The model under review builds one solid part; all positions refer to its coordinate system, in mm. A direction names the side the tool comes from. Coordinates: 2 decimals unless noted, no trailing zeros. Order: outer loops, then holes, each group sorted by start corner. A loop starts at its lowest first (then second) coordinate and runs counter-clockwise, first axis right, second up. Notation, with made-up numbers: M 81,-33.5 L 102,-33.5 A33 cw 102,-4.5 Z; hole C 6.5,67 d4. An arc over 180 degrees is marked long. Answer in a Markdown table with one row per item.
Solid Edge part; units mm, degrees
sketch "Sketch1" plane through (0, 0, 0) normal (0, -1, 0) x (1, 0, 0)
  line L0 (5.1, 0) -> (5.1, 1.5)
  line L1 (5.1, 1.5) -> (11, 1.5)
  line L2 (11, 1.5) -> (11, 5)
  line L3 (11, 5) -> (5.1, 5)
  line L4 (5.1, 5) -> (5.1, 15)
  line L5 (5.1, 15) -> (4, 15)
  line L6 (4, 15) -> (4, 0)
  line L7 (4, 0) -> (5.1, 0)
  dimension "D1" = 5.1
  dimension "D2" = 11
  dimension "D3" = 5.1
revolve "RevolvedProtrusion1" add sketch "Sketch1" angle 360 about axis through (0, 0, 0) along (0, 0, 1)
sketch "Sketch2" plane through (0, 0, 5) normal (0, 0, 1) x (1, 0, 0)
  circle A0 centre (0, 8) radius 1.6
  circle A1 centre (8, 0) radius 1.6
  circle A2 centre (0, -8) radius 1.6
  circle A3 centre (-8, 0) radius 1.6
extrude "Cutout1" cut sketch "Sketch2" against normal through all
chamfer "Chamfer1" distance 0.4 angle 45 2 edges at (-5.1, 0, 15) (-5.1, 0, 0)
(1) Take a section at A-A (x = 0). Write out the cut boundary in (y, z), then the cut area to 3 significant figures.
Report:
| item | result |
|---|---|
| outline | M -11,1.5 L -9.6,1.5 L -9.6,5 L -11,5 Z; M -6.4,1.5 L -5.1,1.5 L -5.1,0.4 L -4.7,0 L -4,0 L -4,15 L -4.7,15 L -5.1,14.6 L -5.1,5 L -6.4,5 Z; M 4,0 L 4.7,0 L 5.1,0.4 L 5.1,1.5 L 6.4,1.5 L 6.4,5 L 5.1,5 L 5.1,14.6 L 4.7,15 L 4,15 Z; M 9.6,1.5 L 11,1.5 L 11,5 L 9.6,5 Z |
| area | 51.6 mm^2 |
(2) Take a section at D-D (y = 8). Write out the cut boundary in (x, z).
Report:
| item | result |
|---|---|
| outline | M -7.55,1.5 L -1.6,1.5 L -1.6,5 L -7.55,5 Z; M 1.6,1.5 L 7.55,1.5 L 7.55,5 L 1.6,5 Z |
(3) The part is to be moulded in two halves that separate along Y. For faces 3 (the cylindrical face through (-9.6, 0.07, 3.27)), 4 (the cylindrical face through (2.4, -4.5, 9.9)), 5 (the flat face through (2, -5, 5)), say which applies: +Y half, -Y half, draft (parallel to the pull), parting line (faces both ways), or undercut.
Report:
| item | result |
|---|---|
| face 3 | undercut |
| face 4 | parting line |
| face 5 | draft |
(4) Insertion check: P1, Ø5, axis at x = 8, y = 0, coming from the -Z side; P2, Ø4, axis at x = -5.5, z = 2, coming from the +Y side; P3, Ø1.9, axis at x = 0, y = 8, coming from the +Z side; P4, Ø5, axis at x = -8, y = 0, coming from the +Z side. Each pin has a flat end and moves straight along its axis. Give the tip position at first contact, or say it passes through.
Report:
| item | result |
|---|---|
| P1 | z = 1.5 |
| P2 | y = 10.43 |
| P3 | through |
| P4 | z = 5 |
(5) Machinability: for faces 1 (the cylindrical face through (-0.35, -9.56, 3.27)), 2 (the flat face through (2, -5, 1.5)), which of the approach directions +Z, -Z, +X, -X, +Y, -Y give a long, thin tool a straight path to every point of the face, cutting with its end or side? Answer none if there is none.
Report:
| item | result |
|---|---|
| face 1 | +Z, -Z |
| face 2 | -Z |
(6) Take a section at C-C (z = 4.5). Write out the cut boundary in (x, y).
Report:
| item | result |
|---|---|
| outline | C 0,0 d22; hole C -8,0 d3.2; hole C 0,0 d8; hole C 0,-8 d3.2; hole C 0,8 d3.2; hole C 8,0 d3.2 |
(7) To check wall thickness, follow line 1 (Y direction, x = 0, z = 4.2); line 2 (Y direction, x = 0, z = 6.25); line 3 (X direction, y = -1, z = 2). State the ranges of each line that lie inside material, in increasing order. Write a range as [from, to].
Report:
| item | result |
|---|---|
| line 1 | [-11, -9.6], [-6.4, -4], [4, 6.4], [9.6, 11] |
| line 2 | [-5.1, -4], [4, 5.1] |
| line 3 | [-10.95, -9.25], [-6.75, -3.87], [3.87, 6.75], [9.25, 10.95] |
